For this review, take the finished solid that the model builds, in its own axes (mm). A direction names the side the tool comes from. Give positions to 0.01 mm unless a question says otherwise; leave off trailing zeros. Order: outer loops, then holes, each group sorted by start corner. A loop starts at its lowest first (then second) coordinate and runs counter-clockwise, first axis right, second up.
from build123d import *

# Parameters (mm, degrees)
SALIENTE_EXTRUIR1_DEPTH = 10


with BuildPart() as part:
    # Croquis1 → Saliente-Extruir1 (new body)
    with BuildSketch(Plane(origin=(0, 0, 0), x_dir=(0, 1, 0), z_dir=(0, 0, 1))):
        Polygon((3.05, 8.067721178), (0, 8.067721178), (0, 0), (3.05, 4.767721178), align=None)
        Polygon((-3.05, 10.867721178), (-3.05, 8.067721178), (0, 8.067721178), (3.05, 8.067721178), (3.05, 10.867721178), align=None)
    extrude(amount=SALIENTE_EXTRUIR1_DEPTH)


solid = part.part
1) We need section C-C on x = -5.25. Give the boundary of the cut face in (y, z).
Answer sheet:
outline: (0, 0) - (3.05, 0) - (3.05, 10) - (0, 10) - close
2) Clearance check with flat-ended pins moving along their axes: pin 1 (3 mm diameter, centred on x = -3.5, y = -0.5, fed in from -Z); pin 2 (3 mm diameter, centred on x = -3, z = 1, fed in from +Y); pin 3 (3.5 mm diameter, centred on y = -2, z = 4, fed in from +X); pin 4 (4 mm diameter, centred on x = -4, z = 7.5, fed in from -Y). State where each tip first meets the part, or that it passes through.
Answer sheet:
pin 1: stops at z = 0
pin 2: stops at y = 2.88
pin 3: stops at x = -8.07
pin 4: stops at y = 0
3) Tool access review of faces 4 (the face through (-8.068, -2, 5)), 5 (the face through (-8, 1, 0)): name each direction out of +Z, -Z, +X, -X, +Y, -Y from which nothing blocks a thin tool from reaching the whole face with its end or side.
Answer sheet:
face 4: +Z, -Z, +X, -Y
face 5: -Z, +X, -X, +Y, -Y
4) We need section A-A on z = 1.75. Give the boundary of the cut face in (x, y), then the cut area to 3 significant figures.
Answer sheet:
outline: (-10.87, -3.05) - (-8.07, -3.05) - (-8.07, 0) - (0, 0) - (-4.77, 3.05) - (-10.87, 3.05) - close
area: 34.4 mm2
5) We need section B-B on y = -2. Give the boundary of the cut face in (x, z).
Answer sheet:
outline: (-10.87, 0) - (-8.07, 0) - (-8.07, 10) - (-10.87, 10) - close
6) Draft analysis for pull direction X (two halves, no side actions). For faces 1 (the face through (-10.868, 0, 5)), 2 (the face through (-2.35, 1.504, 4.93)), 3 (the face through (-4, 0, 5)), state which applies: +X half, -X half, draft (parallel to the pull), parting line (faces both ways), or undercut.
Answer sheet:
face 1: -X half
face 2: +X half
face 3: draft
7) To check wall thickness, follow line 1 (Y direction, x = -8, z = 8); line 2 (X direction, y = -1.5, z = 2.5); line 3 (Y direction, x = -2, z = 4.75). State the ranges of each line that lie inside material, in increasing order.
Answer sheet:
line 1: y = 0 to 3.05
line 2: x = -10.87 to -8.07
line 3: y = 0 to 1.28
